from build123d import *

# Parameters (mm, degrees)
SKETCH3_W                = 38.1
SKETCH3_H                = 38.1
SKETCH3_W_2              = 32.004
SKETCH3_H_2              = 32.004
BOSS_EXTRUDE1_DEPTH      = 1219.2
BOSS_EXTRUDE1_DEPTH_BACK = 1219.2
FILLET1_R                = 1.524
FILLET2_R                = 0.3048


with BuildPart() as part:
    # Sketch3 → Boss-Extrude1 (new body, two sides)
    with BuildSketch(Plane.XY) as boss_extrude1_sk:
        Rectangle(SKETCH3_W, SKETCH3_H)
        Rectangle(SKETCH3_W_2, SKETCH3_H_2, mode=Mode.SUBTRACT)
    extrude(amount=BOSS_EXTRUDE1_DEPTH)
    extrude(boss_extrude1_sk.sketch, amount=-BOSS_EXTRUDE1_DEPTH_BACK)

    # Fillet1
    fillet1_edges = [part.edges().sort_by_distance(p)[0] for p in [
        (-19.05, -19.05, 0),
        (-19.05, 19.05, 0),
        (19.05, 19.05, 0),
        (19.05, -19.05, 0),
    ]]
    fillet(fillet1_edges, radius=FILLET1_R)

    # Fillet2
    fillet2_edges = [part.edges().sort_by_distance(p)[0] for p in [
        (-16.002, -16.002, 0),
        (16.002, -16.002, 0),
        (16.002, 16.002, 0),
        (-16.002, 16.002, 0),
    ]]
    fillet(fillet2_edges, radius=FILLET2_R)


solid = part.part
Here's how the part is built. I have some questions about the finished solid (model axes, mm). Coordinates: 2 decimals unless noted, no trailing zeros. Loops run counter-clockwise (first coordinate to the right, second up) from the corner with the lowest first, then second, coordinate; pieces in that order, holes last. Notation, with made-up numbers: (85, -23.5) -> (133, -23.5) arc R11 cw to (133, -16.5) -> close; hole circle Ø3 at (22, 82). An arc over 180 degrees is marked (long way). Use one line per item in the form item = value. Start each with the question number.
(1) If we section it at C-C (z = 559): Please give me the cut outline in (x, y), then the cut area to 3 significant figures.
(2) If we section it at A-A (x = 2.5): Please give me the cut outline in (y, z).
(3) Please list where this line runs through material, in increasing order: line 1 along Y through (x, z) = (14, -44).
Verdict:
q1.outline = (-19.05, -17.53) arc R1.52 ccw to (-17.53, -19.05) -> (17.53, -19.05) arc R1.52 ccw to (19.05, -17.53) -> (19.05, 17.53) arc R1.52 ccw to (17.53, 19.05) -> (-17.53, 19.05) arc R1.52 ccw to (-19.05, 17.53) -> close; hole (-16, -15.7) arc R0.3 ccw to (-15.7, -16) -> (15.7, -16) arc R0.3 ccw to (16, -15.7) -> (16, 15.7) arc R0.3 ccw to (15.7, 16) -> (-15.7, 16) arc R0.3 ccw to (-16, 15.7) -> close
q1.area = 425 mm²
q2.outline = (-19.05, -1219.2) -> (-16, -1219.2) -> (-16, 1219.2) -> (-19.05, 1219.2) -> close; (16, -1219.2) -> (19.05, -1219.2) -> (19.05, 1219.2) -> (16, 1219.2) -> close
q3.line_1 = -19.05 to -16, 16 to 19.05
